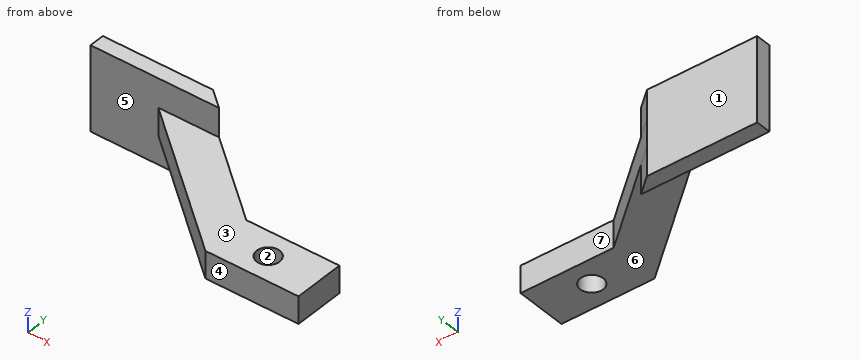
```python
from build123d import *

# Parameters (mm, degrees)
SZKIC1_W                    = 55
SZKIC1_H                    = 30
SZKIC1_R                    = 6.75
DODANIE_WYCI_GNI_CIE1_DEPTH = 8
DODANIE_WYCI_GNI_CIE2_DEPTH = 25


with BuildPart() as part:
    # Szkic1 → Dodanie-wyciągnięcie1 (new, symmetric)
    # profile 1 of 2: a face of its own
    with BuildSketch(Plane.XY):
        with Locations((-27.5, -15)):
            Rectangle(SZKIC1_W, SZKIC1_H)
        with Locations((-30, -15)):
            Circle(SZKIC1_R, mode=Mode.SUBTRACT)
    # profile 2 of 2: a face of its own
    with BuildSketch(Plane.XY):
        Polygon((-114.85915493, 50), (-55, 0), (-55, -30), (-140, 41), (-180, 41), (-180, 50), align=None)
    extrude(amount=DODANIE_WYCI_GNI_CIE1_DEPTH, both=True)

    # Szkic2 → Dodanie-wyciągnięcie2 (add, symmetric)
    with BuildSketch(Plane.XY):
        Polygon((-180, 41), (-140, 41), (-104.084507042, 41), (-114.85915493, 50), (-180, 50), align=None)
    extrude(amount=DODANIE_WYCI_GNI_CIE2_DEPTH, both=True)


solid = part.part
```
Work out the finished part from the listing and answer in its coordinate system (mm). Face numbers are marked on the shaded views. A direction names the side the tool comes from. Give positions to 0.01 mm unless a question says otherwise; leave off trailing zeros. Order: outer loops, then holes, each group sorted by start corner. A loop starts at its lowest first (then second) coordinate and runs counter-clockwise, first axis right, second up. Notation, with made-up numbers: (77.25, -22) -> (105.25, -22) arc R30 ccw to (105.25, 1) -> close; hole circle Ø5 at (-19, 67). An arc over 180 degrees is marked (long way). Answer as CSV lines item,"result". Start each with the question number.
(1) Section D-D, the plane z = 20.5 is taken. Write down the section's boundary in (x, y).
(2) Each of these flat-tipped pins is pushed along its axis until it touches: pin 1 Ø1 at (x, y) = (-61.5, 5) entering from -Z; pin 2 Ø12 at (x, y) = (-84, 0.5) entering from +Z; pin 3 Ø8 at (y, z) = (4.5, 6) entering from -X. Where does it stop, or does it pass through?
(3) Consider line 1 along Y through (x, z) = (-30, 3.5); line 2 along Y through (x, z) = (-134.5, -12); line 3 along Z through (x, y) = (-75, 4.5). Determine where each line is inside the solid, lowest interval first.
(4) Which of the six approach directions +Z, -Z, +X, -X, +Y, -Y give full straight-line access (tool end or side, diameter ignored) to the marked faces 4, 5, 6 and 7?
(5) Section C-C, the plane x = -118.5 is taken. Write down the section's boundary in (y, z).
(6) Section B-B, the plane y = -15 is taken. Write down the section's boundary in (x, z), plus the area to 3 significant figures.
(7) Section A-A, the plane x = -30 is taken. Write down the section's boundary in (y, z).
(8) For a pull along Y with two mould halves and no side action, classify the marked faces 1, 2 and 3 as released by +Y, released by -Y, zero draft, split by the parting line, or undercut.
Entries:
1,outline,"(-180, 41) -> (-104.08, 41) -> (-114.86, 50) -> (-180, 50) -> close"
2,pin 1,"z = -8"
2,pin 2,"z = 8"
2,pin 3,"x = -101.09"
3,line 1,"-30 to -21.75, -8.25 to 0"
3,line 2,"41 to 50"
3,line 3,"-8 to 8"
4,face 4,"+Z, -Z, +X, -X, -Y"
4,face 5,"-X, -Y"
4,face 6,"-Z, +X, -X, -Y"
4,face 7,"+Z, -Z, +X, +Y"
5,outline,"(23.04, -8) -> (41, -8) -> (41, -25) -> (50, -25) -> (50, 25) -> (41, 25) -> (41, 8) -> (23.04, 8) -> close"
6,outline,"(-72.96, -8) -> (-36.75, -8) -> (-36.75, 8) -> (-72.96, 8) -> close; (-23.25, -8) -> (0, -8) -> (0, 8) -> (-23.25, 8) -> close"
6,area,"951 mm²"
7,outline,"(-30, -8) -> (-21.75, -8) -> (-21.75, 8) -> (-30, 8) -> close; (-8.25, -8) -> (0, -8) -> (0, 8) -> (-8.25, 8) -> close"
8,face 1,"released by +Y"
8,face 2,"undercut"
8,face 3,"zero draft"
